For this review, take the finished solid that the model builds, in its own axes (mm). Face numbers are marked on the shaded views. A direction names the side the tool comes from. Round coordinates to 2 decimals unless told otherwise and drop trailing zeros. Loops run counter-clockwise (first coordinate to the right, second up) from the corner with the lowest first, then second, coordinate; pieces in that order, holes last.
1) Take a section at B-B (y = -4). State the section outline as (x, z) points.
2) Wall thickness on L1, parallel to Y at x = 78, z = 11.5; L2, parallel to Y at x = -6.2, z = 18.7; L3, parallel to Y at x = 68, z = 1.75: over which ranges is each line inside the solid? List them lowest first.
3) Tool access review of the marked faces 1, 2, 3, 4 and 5: name each direction out of +Z, -Z, +X, -X, +Y, -Y from which nothing blocks a thin tool from reaching the whole face with its end or side.
4) Mouldability with a two-part tool opening along X and no side actions: class the marked faces 6, 7 and 8 as pulls with the +X half, pulls with the -X half, needs draft (parallel to the pull), parting line crosses it, or undercut.
5) Take a section at D-D (z = 18). Give the number of separate pieces and of enclosed holes in the cut face, then the cut area to 3 significant figures.
6) Insertion check: pin 1 (3 mm diameter, centred on x = -16, z = 9.8, fed in from +Y); pin 2 (4 mm diameter, centred on x = 16, z = 9.8, fed in from +Y). Each pin has a flat end and moves straight along its axis. Give the tip position at first contact, or say it passes through.
7) Take a section at C-C (x = 16). State the section outline as (y, z) points, then the cut area to 3 significant figures.
8) Take a section at A-A (x = 78). State the section outline as (y, z) points, then the cut area to 3 significant figures.
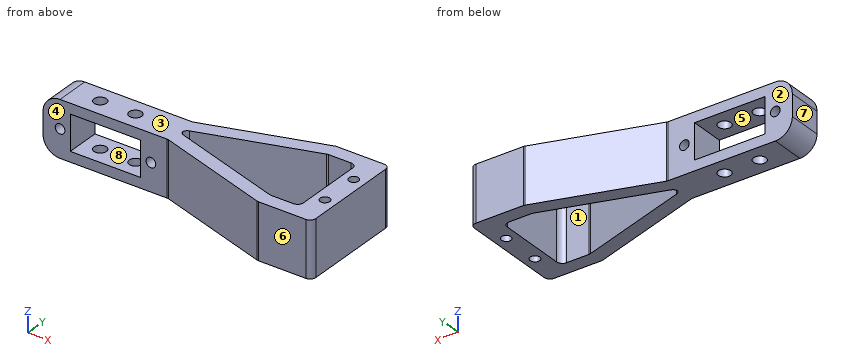
```python
from build123d import *

# Parameters (mm, degrees)
SKETCH_1_R          = 2.2
SKETCH_1_R_2        = 1.7
EXTRUDE_1_DEPTH     = 19.6
SKETCH_2_R          = 1.7
SKETCH_2_W          = 24.8
SKETCH_2_H          = 12.4
CUT_EXTRUDE_1_DEPTH = 88.938387522
CUT_EXTRUDE_2_DEPTH = 87.424302138
FILLET_1_R          = 2
FILLET_2_R          = 6


with BuildPart() as part:
    # 草图1 → 凸台-拉伸1 (new body)
    with BuildSketch(Plane.XY):
        Polygon((-22, -6), (22, -6), (63, -19), (82, -19), (82, 19), (63, 19), (22, 6), (-22, 6), align=None)
        with Locations((-6.2, 0)):
            Circle(SKETCH_1_R, mode=Mode.SUBTRACT)
        with Locations((6.2, 0)):
            Circle(SKETCH_1_R, mode=Mode.SUBTRACT)
        with Locations((78, 7)):
            Circle(SKETCH_1_R_2, mode=Mode.SUBTRACT)
        with Locations((78, -7)):
            Circle(SKETCH_1_R_2, mode=Mode.SUBTRACT)
    extrude(amount=EXTRUDE_1_DEPTH)

    # 草图2 → 切除-拉伸1 (cut, through all)
    with BuildSketch(Plane(origin=(0, 6, 0), x_dir=(1, 0, 0), z_dir=(0, 1, 0))):
        with Locations(Location((16, -9.8, 0), (0, 0, 270))):
            Circle(SKETCH_2_R)
        with Locations(Location((-16, -9.8, 0), (0, 0, 270))):
            Circle(SKETCH_2_R)
        with Locations((0, -9.8)):
            Rectangle(SKETCH_2_W, SKETCH_2_H)
    extrude(amount=-CUT_EXTRUDE_1_DEPTH, mode=Mode.SUBTRACT)

    # 草图3 → 切除-拉伸2 (cut, through all)
    with BuildSketch(Plane.XY.offset(19.6)):
        Polygon((74, 14), (74, -14), (63.773702437, -14), (22.773702437, -1), (22.773702437, 1), (63.773702437, 14), align=None)
    extrude(amount=-CUT_EXTRUDE_2_DEPTH, mode=Mode.SUBTRACT)

    # 圆角1
    # the kernel refuses this fillet: 2 mm, written as the material it adds along each edge
    with BuildSketch(Plane(origin=(74, 14, 19.6), x_dir=(-1, 0, 0), z_dir=(0, 0, -1))) as fillet_1_piece_1:
        with BuildLine():
            CenterArc((FILLET_1_R, -FILLET_1_R), FILLET_1_R, 90, 90)
            Line((0, -FILLET_1_R), (0, 0))
            Line((0, 0), (FILLET_1_R, 0))
        make_face()
    extrude(amount=19.6)
    with BuildSketch(Plane(origin=(63.773702437, 14, 19.6), x_dir=(1, 0, 0), z_dir=(0, 0, -1)), Plane(origin=(63.773702437, -14, 19.6), x_dir=(-0.9532306376993169, 0.30224386073393383, 0), z_dir=(0, 0, -1)), Plane(origin=(22, -6, 0), x_dir=(-1, 0, 0), z_dir=(0, 0, 1))) as fillet_1_piece_2:
        with BuildLine():
            CenterArc((FILLET_1_R * 0.154740487324, FILLET_1_R), FILLET_1_R, 252.407575438, 17.592424562)
            Line((-FILLET_1_R * 0.14750337341, FILLET_1_R * 0.0467693623007), (0, 0))
            Line((0, 0), (FILLET_1_R * 0.154740487324, 0))
        make_face()
    extrude(amount=19.6)
    with BuildSketch(Plane(origin=(74, -14, 19.6), x_dir=(-1, 0, 0), z_dir=(0, 0, -1))) as fillet_1_piece_3:
        with BuildLine():
            CenterArc((FILLET_1_R, FILLET_1_R), FILLET_1_R, 180, 90)
            Line((0, FILLET_1_R), (0, 0))
            Line((0, 0), (FILLET_1_R, 0))
        make_face()
    extrude(amount=19.6)
    with BuildSketch(Plane(origin=(22.773702437, 1, 19.6), x_dir=(0.9532306376993182, 0.30224386073392995, 0), z_dir=(0, 0, -1)), Plane(origin=(22.773702437, -1, 19.6), x_dir=(0, 1, 0), z_dir=(0, 0, -1))) as fillet_1_piece_4:
        with BuildLine():
            CenterArc((FILLET_1_R * 0.731990886225, FILLET_1_R), FILLET_1_R, 197.592424562, 72.407575438)
            Line((-FILLET_1_R * 0.221239751475, FILLET_1_R * 0.697756139266), (0, 0))
            Line((0, 0), (FILLET_1_R * 0.731990886225, 0))
        make_face()
    extrude(amount=19.6)
    with BuildSketch(Plane(origin=(22, 6, 0), x_dir=(-1, 0, 0), z_dir=(0, 0, 1))) as fillet_1_piece_5:
        with BuildLine():
            CenterArc((FILLET_1_R * 0.154740487324, -FILLET_1_R), FILLET_1_R, 90, 17.592424562)
            Line((-FILLET_1_R * 0.14750337341, -FILLET_1_R * 0.0467693623007), (0, 0))
            Line((0, 0), (FILLET_1_R * 0.154740487324, 0))
        make_face()
    extrude(amount=19.6)
    # the kernel refuses this fillet: 2 mm, written as the material it takes off along each edge
    with BuildSketch(Plane(origin=(82, -19, -5), x_dir=(-1, 0, 0), z_dir=(0, 0, 1)), Plane(origin=(82, 19, -5), x_dir=(0, -1, 0), z_dir=(0, 0, 1))) as fillet_1_2_piece_1:
        with BuildLine():
            CenterArc((FILLET_1_R, -FILLET_1_R), FILLET_1_R, 90, 90)
            Line((0, -FILLET_1_R), (0, 0))
            Line((0, 0), (FILLET_1_R, 0))
        make_face()
    extrude(amount=29.6, mode=Mode.SUBTRACT)
    with BuildSketch(Plane(origin=(63, -19, -0.773702437), x_dir=(-0.9532306376993186, 0.3022438607339286, 0), z_dir=(0, 0, 1))) as fillet_1_2_piece_2:
        with BuildLine():
            CenterArc((FILLET_1_R * 0.154740487324, -FILLET_1_R), FILLET_1_R, 90, 17.592424562)
            Line((-FILLET_1_R * 0.14750337341, -FILLET_1_R * 0.0467693623007), (0, 0))
            Line((0, 0), (FILLET_1_R * 0.154740487324, 0))
        make_face()
    extrude(amount=21.147404873, mode=Mode.SUBTRACT)
    with BuildSketch(Plane(origin=(63, 19, -0.773702437), x_dir=(-0.9532306376993186, -0.3022438607339286, 0), z_dir=(0, 0, 1))) as fillet_1_2_piece_3:
        with BuildLine():
            CenterArc((FILLET_1_R * 0.154740487324, FILLET_1_R), FILLET_1_R, 252.407575438, 17.592424562)
            Line((-FILLET_1_R * 0.14750337341, FILLET_1_R * 0.0467693623007), (0, 0))
            Line((0, 0), (FILLET_1_R * 0.154740487324, 0))
        make_face()
    extrude(amount=21.147404873, mode=Mode.SUBTRACT)

    # 圆角2
    fillet_2_edges = [part.edges().sort_by_distance(p)[0] for p in [
        (-22, 0, 0),
        (-22, 0, 19.6),
    ]]
    fillet(fillet_2_edges, radius=FILLET_2_R)


solid = part.part
```
Response:
1. outline: (-22, 6) arc R6 ccw to (-16, 0) - (32.24, 0) - (32.24, 19.6) - (-16, 19.6) arc R6 ccw to (-22, 13.6) - close; (74, 0) - (82, 0) - (82, 19.6) - (74, 19.6) - close; hole circle Ø3.4 at (-16, 9.8); hole (-12.4, 3.6) - (12.4, 3.6) - (12.4, 16) - (-12.4, 16) - close; hole circle Ø3.4 at (16, 9.8)
2. L1: y = -19 to -8.7, -5.3 to 5.3, 8.7 to 19
2. L2: y = -6 to -2.2, 2.2 to 6
2. L3: y = -19 to -14, 14 to 19
3. face 1: +Z, -Z
3. face 2: +Z, -Z, -X, +Y
3. face 3: +Z, +X, -X, +Y, -Y
3. face 4: +Z, -Z, -X, -Y
3. face 5: +Y, -Y
4. face 6: needs draft
4. face 7: pulls with the -X half
4. face 8: undercut
5. separate pieces: 1
5. enclosed holes: 5
5. area: 1,300 mm2
6. pin 1: passes through
6. pin 2: stops at y = 6
7. outline: (-6, 0) - (6, 0) - (6, 8.1) - (-6, 8.1) - close; (-6, 11.5) - (6, 11.5) - (6, 19.6) - (-6, 19.6) - close
7. area: 194 mm2
8. outline: (-19, 0) - (-8.7, 0) - (-8.7, 19.6) - (-19, 19.6) - close; (-5.3, 0) - (5.3, 0) - (5.3, 19.6) - (-5.3, 19.6) - close; (8.7, 0) - (19, 0) - (19, 19.6) - (8.7, 19.6) - close
8. area: 612 mm2
